Check sheet for the modelled part. Datum: model origin and axes. Units: mm. A direction names the side the tool comes from. Coordinates: 2 decimals unless noted, no trailing zeros. Loops run counter-clockwise (first coordinate to the right, second up) from the corner with the lowest first, then second, coordinate; pieces in that order, holes last.
```python
from build123d import *

# Parameters (mm, degrees)
SKETCH_W     = 80
SKETCH_H     = 20
PAD_DEPTH    = 6
POCKET_DEPTH = 4


with BuildPart() as part:
    # Sketch → Pad (new body)
    with BuildSketch(Plane.XY):
        Rectangle(SKETCH_W, SKETCH_H)
    extrude(amount=PAD_DEPTH)

    # Sketch001 → Pocket (cut)
    with BuildSketch(Plane.XY.offset(6)):
        with BuildLine():
            ThreePointArc((-31.3, 2.8), (-34.1, 0), (-31.3, -2.8))
            Line((-31.3, -2.8), (-28.5, -2.8))
            ThreePointArc((-28.5, -2.8), (-25.7, 0), (-28.5, 2.8))
            Line((-31.3, 2.8), (-28.5, 2.8))
        make_face()
    extrude(amount=-POCKET_DEPTH, mode=Mode.SUBTRACT)


solid = part.part
```
1) Set-up check for faces 4 (the flat face through (-30, 2.8, 4)), 5 (the flat face through (-40, 0, 3)): record each of +Z, -Z, +X, -X, +Y, -Y from which the full face is reachable in a straight line by a thin tool's end or side.
Answer sheet:
face 4: +Z
face 5: +Z, -Z, -X, +Y, -Y
2) Mould release check, pull along Y, two halves, no side actions. Record for faces 1 (the flat face through (-1, 0, 0)), 2 (the cylindrical face through (-34.1, 0.1, 4)), 3 (the flat face through (-1, -10, 3)): +Y half, -Y half, draft (parallel to the pull), parting line (faces both ways), or undercut.
Answer sheet:
face 1: draft
face 2: undercut
face 3: -Y half
3) Depth check by flat-ended pin: pin 1 (3 mm diameter, centred on x = -28.5, y = 1, fed in from +Z). Enter the tip coordinate at first touch or a pass-through.
Answer sheet:
pin 1: stops at z = 2
4) Section check A-A on y = 0. Enter the section's corners in (x, z).
Answer sheet:
outline: (-40, 0) - (40, 0) - (40, 6) - (-25.7, 6) - (-25.7, 2) - (-34.1, 2) - (-34.1, 6) - (-40, 6) - close
5) Scan lines: line 1 (X direction, y = 0.25, z = 4.3); line 2 (X direction, y = -1.25, z = 3.15). Record each from-to range of solid material in increasing order.
Answer sheet:
line 1: x = -40 to -34.09, -25.71 to 40
line 2: x = -40 to -33.81, -25.99 to 40
